The figure shows three views and two pictorial views of one solid part (mm, origin at its lowest corner). Answer the questions. A direction names the side the tool comes from. Give positions to 0.01 mm unless a question says otherwise; leave off trailing zeros. Order: outer loops, then holes, each group sorted by start corner. A loop starts at its lowest first (then second) coordinate and runs counter-clockwise, first axis right, second up. Notation, with made-up numbers: (21, 73) - (80, 73) arc R33 cw to (80, 105) - close; hole circle Ø11 at (-12, 74). An arc over 180 degrees is marked (long way). Answer as a JSON object with one key per item and string values. Group by question number.
Q1. The mould has two halves that part along X. Classify the marked faces 1, 2 and 3: released by +X, released by -X, zero draft, split by the parting line, or undercut.
Q2. A cutting plane is placed at D-D, the plane z = 12.5. Give the vertices of the cut face in (x, y).
Q3. For the marked faces 4 and 5, determine the directions among +Z, -Z, +X, -X, +Y, -Y from which every point of the face is accessible in a straight line to the end or side of a thin tool.
Q4. Given pin 1 (1.1 mm diameter, centred on x = 35.5, z = 38.5, fed in from -Y); pin 2 (4 mm diameter, centred on y = 9.5, z = 13, fed in from -X); pin 3 (3.5 mm diameter, centred on x = 1.5, z = 25.5, fed in from +Y), each flat-ended and moving along its own axis, determine where each tip first touches the part or whether it passes through.
Q5. A cutting plane is placed at A-A, the plane y = 2.5. Give the vertices of the cut face in (x, z), and give its area (3 significant figures).
Q6. Consider line 1 (X direction, y = 7, z = 35.5); line 2 (X direction, y = 9.5, z = 5); line 3 (X direction, y = 12, z = 12.5). Determine where each line is inside the solid, lowest interval first.
Q7. A cutting plane is placed at C-C, the plane x = 4.5. Give the vertices of the cut face in (y, z), and give its area (3 significant figures).
Q8. A cutting plane is placed at B-B, the plane z = 35.5. Give the vertices of the cut face in (x, y).
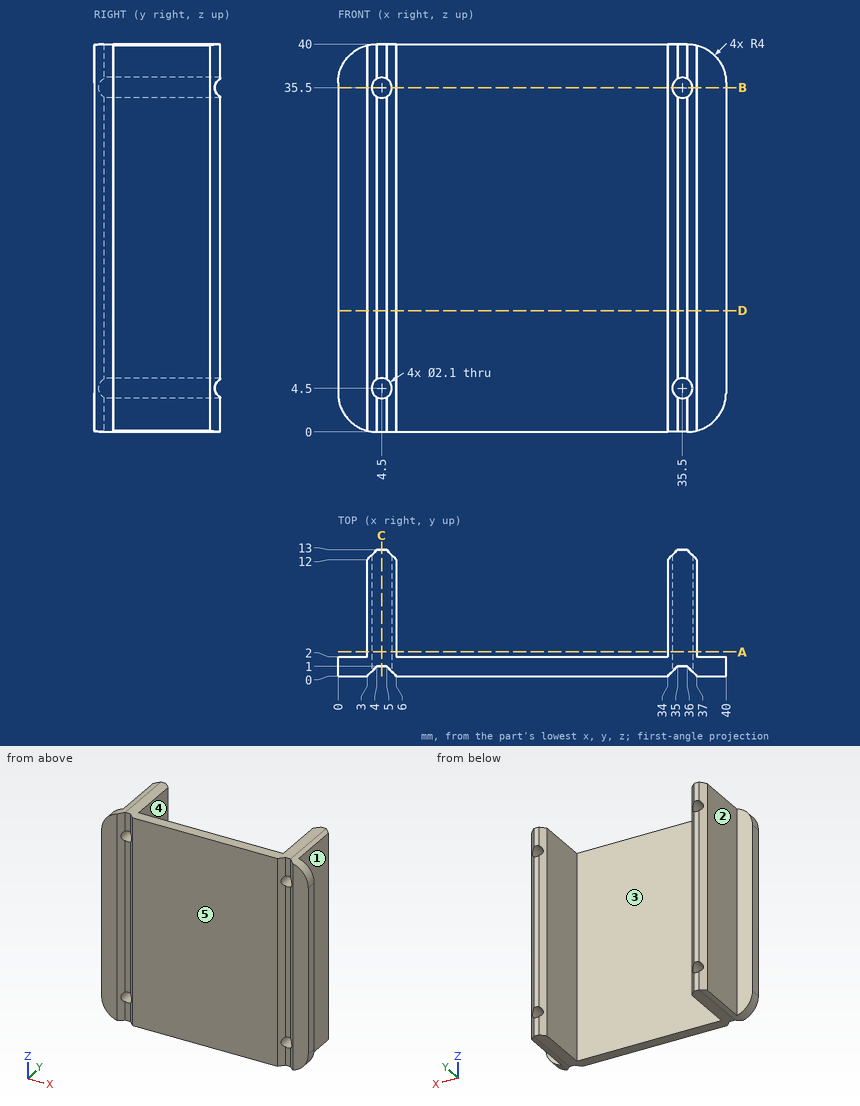
Reply:
{
 "1": {"face 1": "released by +X", "face 2": "released by -X", "face 3": "undercut"},
 "2": {"outline": "(0, 0) - (3, 0) - (4, 1) - (5, 1) - (6, 0) - (34, 0) - (35, 1) - (36, 1) - (37, 0) - (40, 0) - (40, 2) - (37, 2) - (37, 12) - (36, 13) - (35, 13) - (34, 12) - (34, 2) - (6, 2) - (6, 12) - (5, 13) - (4, 13) - (3, 12) - (3, 2) - (0, 2) - close"},
 "3": {"face 4": "+Z, -Z, +Y", "face 5": "+Z, -Z, +X, -X, -Y"},
 "4": {"pin 1": "stops at y = 0.95", "pin 2": "stops at x = 3", "pin 3": "stops at y = 12.25"},
 "5": {"outline": "(3, 0.13) arc R4 ccw to (4, 0) - (6, 0) - (6, 40) - (4, 40) arc R4 ccw to (3, 39.87) - close; (34, 0) - (36, 0) arc R4 ccw to (37, 0.13) - (37, 39.87) arc R4 ccw to (36, 40) - (34, 40) - close; hole circle Ø2.1 at (4.5, 4.5); hole circle Ø2.1 at (4.5, 35.5); hole circle Ø2.1 at (35.5, 4.5); hole circle Ø2.1 at (35.5, 35.5)", "area": "226 mm^2"},
 "6": {"line 1": "x = 3 to 3.45, 5.55 to 6, 34 to 34.45, 36.55 to 37", "line 2": "x = 3 to 3.58, 5.42 to 6, 34 to 34.58, 36.42 to 37", "line 3": "x = 3 to 6, 34 to 37"},
 "7": {"outline": "(1, 0) - (13, 0) - (13, 3.45) - (1, 3.45) - close; (1, 5.55) - (13, 5.55) - (13, 34.45) - (1, 34.45) - close; (1, 36.55) - (13, 36.55) - (13, 40) - (1, 40) - close", "area": "430 mm^2"},
 "8": {"outline": "(0, 0) - (3, 0) - (3.45, 0.45) - (3.45, 12.45) - (3, 12) - (3, 2) - (0, 2) - close; (5.55, 0.45) - (6, 0) - (34, 0) - (34.45, 0.45) - (34.45, 12.45) - (34, 12) - (34, 2) - (6, 2) - (6, 12) - (5.55, 12.45) - close; (36.55, 0.45) - (37, 0) - (40, 0) - (40, 2) - (37, 2) - (37, 12) - (36.55, 12.45) - close"}
}
